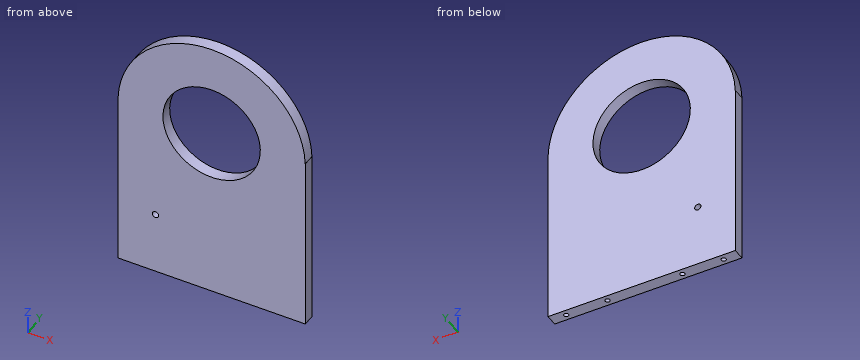
```python
from build123d import *

# Parameters (mm, degrees)
PARED_START                = 29.75
SK_PARED_W                 = 100
SK_PARED_H                 = 95.3
PARED_DEPTH                = 6.35
CABEZA_START               = 29.75
SK_CABEZA_R                = 50
CABEZA_DEPTH               = 6.35
PASO_CUBO_J2_START         = 29.75
SK_PASO_CUBO_J2_R          = 26
PASO_CUBO_J2_DEPTH         = 6.35
PASANTE_M3_CINCHO_START    = 29.75
SK_PASANTE_M3_CINCHO_R     = 1.7
PASANTE_M3_CINCHO_DEPTH    = 6.35
SK_ROSCA_M3_DESDE_ABAJO_R  = 1.25
ROSCA_M3_DESDE_ABAJO_DEPTH = 9


with BuildPart() as part:
    # Sk_Pared → Pared (new body)
    with BuildSketch(Plane(origin=(0, 0, 0), x_dir=(1, 0, 0), z_dir=(0, 1, 0)).offset(PARED_START)):
        with Locations((0, -124)):
            Rectangle(SK_PARED_W, SK_PARED_H)
    extrude(amount=PARED_DEPTH)

    # Sk_Cabeza → Cabeza (add)
    with BuildSketch(Plane(origin=(0, 0, 0), x_dir=(1, 0, 0), z_dir=(0, 1, 0)).offset(CABEZA_START)):
        with Locations((0, -170)):
            Circle(SK_CABEZA_R)
    extrude(amount=CABEZA_DEPTH)

    # Sk_Paso_cubo_J2 → Paso_cubo_J2 (cut)
    with BuildSketch(Plane(origin=(0, 0, 0), x_dir=(1, 0, 0), z_dir=(0, 1, 0)).offset(PASO_CUBO_J2_START)):
        with Locations(Location((0, -170, 0), (0, 0, 270))):
            Circle(SK_PASO_CUBO_J2_R)
    extrude(amount=PASO_CUBO_J2_DEPTH, mode=Mode.SUBTRACT)

    # Sk_Pasante_M3_cincho → Pasante_M3_cincho (cut)
    with BuildSketch(Plane(origin=(0, 0, 0), x_dir=(1, 0, 0), z_dir=(0, 1, 0)).offset(PASANTE_M3_CINCHO_START)):
        with Locations(Location((-30, -110, 0), (0, 0, 270))):
            Circle(SK_PASANTE_M3_CINCHO_R)
    extrude(amount=PASANTE_M3_CINCHO_DEPTH, mode=Mode.SUBTRACT)

    # Sk_Rosca_M3_desde_abajo → Rosca_M3_desde_abajo (cut)
    with BuildSketch(Plane(origin=(0, 0, 76.35), x_dir=(-1, 0, 0), z_dir=(0, 0, -1))):
        with Locations((42, 32.9275)):
            Circle(SK_ROSCA_M3_DESDE_ABAJO_R)
        with Locations((20, 32.9275)):
            Circle(SK_ROSCA_M3_DESDE_ABAJO_R)
        with Locations((-20, 32.9275)):
            Circle(SK_ROSCA_M3_DESDE_ABAJO_R)
        with Locations((-42, 32.9275)):
            Circle(SK_ROSCA_M3_DESDE_ABAJO_R)
    extrude(amount=-ROSCA_M3_DESDE_ABAJO_DEPTH, mode=Mode.SUBTRACT)


solid = part.part
```
The listing builds one solid part. Answer for the finished solid, in the listing's coordinates (mm). Coordinates: 2 decimals unless noted, no trailing zeros. Write each loop counter-clockwise with the first axis right and the second up, starting at its lowest first coordinate (ties: lowest second). Pieces come first, ordered by that corner, then holes. Notation, with made-up numbers: (-38.5, 37) - (-16.5, 37) arc R31 ccw to (-16.5, 71) - close; hole circle Ø3 at (61, 50). An arc over 180 degrees is marked (long way). Return JSON: item names as keys, results as strings. Group by question number.
1. A cutting plane is placed at B-B, the plane x = -12. Determine the outline of the cut face in (y, z), plus the area to 3 significant figures.
2. Straight lines are drawn through the part: L1, parallel to X at y = 32.25, z = 170; L2, parallel to Y at x = -20, z = 83.25; L3, parallel to Z at x = -1, y = 31.5. For each, find the intervals that lie inside material, in ascending order.
3. Given pin 1 (2 mm diameter, centred on x = -30, z = 110, fed in from +Y); pin 2 (1.5 mm diameter, centred on x = 24.5, y = 35, fed in from +Z); pin 3 (0.8 mm diameter, centred on x = 42, y = 32.5, fed in from -Z); pin 4 (3 mm diameter, centred on x = 42, y = 32.93, fed in from +Z), each flat-ended and moving along its own axis, determine where each tip first touches the part or whether it passes through.
4. A cutting plane is placed at D-D, the plane x = 28.5. Determine the outline of the cut face in (y, z), plus the area to 3 significant figures.
5. A cutting plane is placed at C-C, the plane x = -35. Determine the outline of the cut face in (y, z).
6. A cutting plane is placed at A-A, the plane z = 110. Determine the outline of the cut face in (x, y).
Ans:
{
 "1": {"outline": "(29.75, 76.35) - (36.1, 76.35) - (36.1, 146.93) - (29.75, 146.93) - close; (29.75, 193.07) - (36.1, 193.07) - (36.1, 218.54) - (29.75, 218.54) - close", "area": "610 mm²"},
 "2": {"L1": "-50 to -26, 26 to 50", "L2": "29.75 to 31.68, 34.18 to 36.1", "L3": "76.35 to 144.02, 195.98 to 219.99"},
 "3": {"pin 1": "through", "pin 2": "z = 214", "pin 3": "z = 85.35", "pin 4": "z = 199.32"},
 "4": {"outline": "(29.75, 76.35) - (36.1, 76.35) - (36.1, 211.08) - (29.75, 211.08) - close", "area": "856 mm²"},
 "5": {"outline": "(29.75, 76.35) - (36.1, 76.35) - (36.1, 205.71) - (29.75, 205.71) - close"},
 "6": {"outline": "(-50, 29.75) - (-31.7, 29.75) - (-31.7, 36.1) - (-50, 36.1) - close; (-28.3, 29.75) - (50, 29.75) - (50, 36.1) - (-28.3, 36.1) - close"}
}
